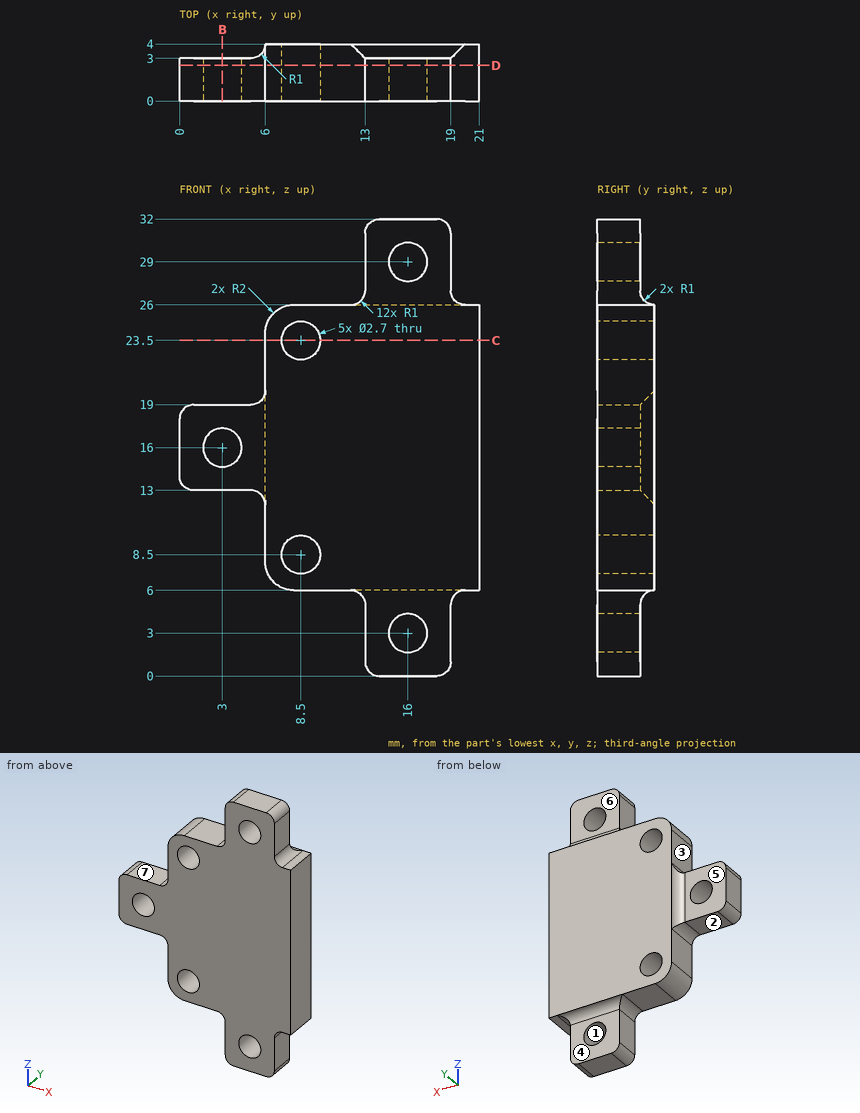
Answer from the drawing. Dimensions are ordinates in mm from the lowest x, y and z of the part. A direction names the side the tool comes from. Coordinates: 2 decimals unless noted, no trailing zeros. Write each loop counter-clockwise with the first axis right and the second up, starting at its lowest first coordinate (ties: lowest second). Pieces come first, ordered by that corner, then holes. Notation, with made-up numbers: (-26.5, 74.5) - (-18.5, 74.5) arc R33 ccw to (-18.5, 103.5) - close; hole circle Ø4 at (-4, 63). An arc over 180 degrees is marked (long way). Return JSON: item names as keys, results as strings. Group by question number.
Q1. Find the intervals of material crossed by line 1 along Z through (x, y) = (16, 0.75); line 2 along Z through (x, y) = (3, 0.65); line 3 along Z through (x, y) = (8.25, 1.35), in increasing order. Write a range as [from, to].
Q2. The part is cut by section C-C on z = 23.5. Write down the section's boundary in (x, y).
Q3. The part is cut by section D-D on y = 2.5. State how many separate pieces and enclosed holes the cut face has, and give its area (3 significant figures).
Q4. The part is cut by section B-B on x = 3. Write down the section's boundary in (y, z).
Q5. Which of the six approach directions +Z, -Z, +X, -X, +Y, -Y give full straight-line access (tool end or side, diameter ignored) to the marked faces 4, 5, 6 and 7?
Q6. Flat-ended cylindrical pins translate along their axes: pin 1 Ø1.5 at (x, z) = (8.5, 4) entering from -Y; pin 2 Ø1.5 at (y, z) = (2, 2) entering from +X; pin 3 Ø1.5 at (x, y) = (3, 1) entering from +Z; pin 4 Ø4.5 at (x, z) = (3, 16) entering from +Y. Find the tip coordinate at first contact, or state that the pin passes through.
Q7. For a pull along X with two mould halves and no side action, classify the marked faces 1, 2 and 3 as +X half, -X half, draft (parallel to the pull), parting line (faces both ways), or undercut.
Evaluation:
{
 "1": {"line 1": "z = [0, 1.65], [4.35, 27.65], [30.35, 32]", "line 2": "z = [13, 14.65], [17.35, 19]", "line 3": "z = [6, 7.17], [9.83, 22.17], [24.83, 26]"},
 "2": {"outline": "(6, 0) - (7.15, 0) - (7.15, 4) - (6, 4) - close; (9.85, 0) - (21, 0) - (21, 4) - (9.85, 4) - close"},
 "3": {"separate pieces": "1", "enclosed holes": "5", "area": "378 mm2"},
 "4": {"outline": "(0, 13) - (3, 13) - (3, 14.65) - (0, 14.65) - close; (0, 17.35) - (3, 17.35) - (3, 19) - (0, 19) - close"},
 "5": {"face 4": "-Z, +X, -X, +Y", "face 5": "+Z, -Z, -X, +Y", "face 6": "+Z, +X, -X, +Y", "face 7": "+Z, -X, +Y, -Y"},
 "6": {"pin 1": "passes through", "pin 2": "stops at x = 19", "pin 3": "stops at z = 19", "pin 4": "stops at y = 3.03"},
 "7": {"face 1": "undercut", "face 2": "draft", "face 3": "-X half"}
}
